```python
from build123d import *

# Parameters (mm, degrees)
BOSS_EXTRUDE1_DEPTH = 3.175
CUT_EXTRUDE1_DEPTH  = 223.25
SKETCH4_W           = 6.35
SKETCH4_H           = 25.4
BOSS_EXTRUDE2_DEPTH = 6.35
LPATTERN1_COUNT     = 3
LPATTERN1_PITCH     = 50.8
SKETCH5_W           = 38.1
SKETCH5_H           = 6.35
BOSS_EXTRUDE3_DEPTH = 6.35
FILLET1_R           = 2.54
CUT_EXTRUDE2_DEPTH  = 6.35


with BuildPart() as part:
    # Sketch1 → Boss-Extrude1 (new, symmetric)
    with BuildSketch(Plane.XY):
        Polygon((0, 190.5), (0, 0), (-114.3, 0), align=None)
    extrude(amount=BOSS_EXTRUDE1_DEPTH, both=True)

    # Sketch2 → Cut-Extrude1 (cut, through all)
    with BuildSketch(Plane.XY.offset(3.175)):
        Polygon((-80.654073281, 19.05), (-19.05, 19.05), (-19.05, 121.723455468), align=None)
    extrude(amount=-CUT_EXTRUDE1_DEPTH, mode=Mode.SUBTRACT)

    # Sketch4 → Boss-Extrude2 (add)
    with BuildSketch(Plane(origin=(0, 0, 0), x_dir=(0, 0, -1), z_dir=(1, 0, 0))):
        with Locations((0, 165.1)):
            Rectangle(SKETCH4_W, SKETCH4_H)
    boss_extrude2 = extrude(amount=BOSS_EXTRUDE2_DEPTH)

    # LPattern1: Boss-Extrude2 ×3
    with Locations(*[(0, -i * LPATTERN1_PITCH, 0) for i in range(1, LPATTERN1_COUNT)]):
        add(boss_extrude2)

    # Sketch5 → Boss-Extrude3 (add)
    with BuildSketch(Plane(origin=(0, 0, 0), x_dir=(-1, 0, 0), z_dir=(0, -1, 0))):
        with Locations((53.975, 0)):
            Rectangle(SKETCH5_W, SKETCH5_H)
    extrude(amount=BOSS_EXTRUDE3_DEPTH)

    # Fillet1
    fillet1_edges = [part.edges().sort_by_distance(p)[0] for p in [
        (-80.654073281, 19.05, 0),
        (-19.05, 121.723455468, 0),
        (-19.05, 19.05, 0),
    ]]
    fillet(fillet1_edges, radius=FILLET1_R)

    # Sketch3 → Cut-Extrude2 (cut)
    with BuildSketch(Plane(origin=(0, 0, -3.175), x_dir=(-1, 0, 0), z_dir=(0, 0, -1))):
        Polygon((91.567, 0), (95.758, 0), (95.758, 8.763), (97.0915, 8.763), (97.0915, 11.303), (95.758, 11.303), (95.758, 14.605), (91.567, 14.605), (91.567, 11.303), (90.2335, 11.303), (90.2335, 8.763), (91.567, 8.763), align=None)
        Polygon((15.367, 0), (19.558, 0), (19.558, 8.763), (20.8915, 8.763), (20.8915, 11.303), (19.558, 11.303), (19.558, 14.605), (15.367, 14.605), (15.367, 11.303), (14.0335, 11.303), (14.0335, 8.763), (15.367, 8.763), align=None)
        Polygon((0, 141.7955), (0, 137.6045), (8.763, 137.6045), (8.763, 136.271), (11.303, 136.271), (11.303, 137.6045), (14.605, 137.6045), (14.605, 141.7955), (11.303, 141.7955), (11.303, 143.129), (8.763, 143.129), (8.763, 141.7955), align=None)
        Polygon((0, 27.4955), (0, 23.3045), (8.763, 23.3045), (8.763, 21.971), (11.303, 21.971), (11.303, 23.3045), (14.605, 23.3045), (14.605, 27.4955), (11.303, 27.4955), (11.303, 28.829), (8.763, 28.829), (8.763, 27.4955), align=None)
    extrude(amount=-CUT_EXTRUDE2_DEPTH, mode=Mode.SUBTRACT)


solid = part.part
```
Read the model definition and answer for the solid it produces. Units are mm, in the model's axes. A direction names the side the tool comes from. Coordinates: 2 decimals unless noted, no trailing zeros. Loops run counter-clockwise (first coordinate to the right, second up) from the corner with the lowest first, then second, coordinate; pieces in that order, holes last.
(1) The mould has two halves that part along Y. Classify faces 1 (the face through (3, 177.8, 0)), 2 (the face through (-73.025, -3, 0)), 3 (the face through (-105, 0, 0)), 4 (the face through (0, 89, 0)): released by +Y, released by -Y, zero draft, split by the parting line, or undercut.
Solution:
face 1: released by +Y
face 2: zero draft
face 3: released by -Y
face 4: undercut
(2) The part is cut by section B-B (y = 97.5). Determine the outline of the cut face in (x, z) (3 decimals), and give its area (3 significant figures).
Solution:
outline: (-55.8, -3.175) - (-33.584, -3.175) - (-33.584, 3.175) - (-55.8, 3.175) - close; (-19.05, -3.175) - (0, -3.175) - (0, 3.175) - (-19.05, 3.175) - close
area: 262 mm2
(3) Consider line 1 along Y through (x, z) = (-4, 1.25); line 2 along X through (y, z) = (5, 1.5); line 3 along Y through (x, z) = (-10, 2.5). Determine where each line is inside the solid, lowest interval first.
Solution:
line 1: y = 0 to 23.3, 27.5 to 137.6, 141.8 to 183.83
line 2: x = -111.3 to -95.76, -91.57 to -19.56, -15.37 to 0
line 3: y = 0 to 21.97, 28.83 to 136.27, 143.13 to 173.83
(4) The part is cut by section D-D (x = -81.5). Determine the outline of the cut face in (y, z) (3 decimals), and give its area (3 significant figures).
Solution:
outline: (0, -3.175) - (54.667, -3.175) - (54.667, 3.175) - (0, 3.175) - close
area: 347 mm2
(5) Flat-ended cylindrical pins translate along their axes: pin 1 Ø1.1 at (y, z) = (23, 0.5) entering from -X; pin 2 Ø3 at (x, z) = (-102.5, 0.5) entering from -Y; pin 3 Ø1.7 at (x, z) = (-13, -1.5) entering from +Y. Find the tip coordinate at first contact, or state that the pin passes through.
Solution:
pin 1: stops at x = -100.83
pin 2: stops at y = 0
pin 3: stops at y = 170.25
(6) The part is cut by section A-A (x = -40.5). Determine the outline of the cut face in (y, z) (3 decimals), and give its area (3 significant figures).
Solution:
outline: (-6.35, -3.175) - (19.05, -3.175) - (19.05, 3.175) - (-6.35, 3.175) - close; (85.973, -3.175) - (123, -3.175) - (123, 3.175) - (85.973, 3.175) - close
area: 396 mm2
(7) A tool of negligible diameter and unlimited length cuts with its end or side. For faces 5 (the face through (-54, -6.35, 0)), 6 (the face through (-4, 137.604, 0)), 7 (the face through (-20.957, 115.013, -0.044)), 8 (the face through (-15.367, 4, 0)), 9 (the face through (-8, 0, 0)), from which of +Z, -Z, +X, -X, +Y, -Y can it reach the whole face along a straight path? Write none if from no direction.
Solution:
face 5: +Z, -Z, +X, -X, -Y
face 6: +Z, -Z, +X
face 7: +Z, -Z
face 8: +Z, -Z, -Y
face 9: +Z, -Z, +X, -Y
(8) The part is cut by section C-C (y = 145.5). Determine the outline of the cut face in (x, z) (3 decimals), and give its area (3 significant figures).
Solution:
outline: (-27, -3.175) - (0, -3.175) - (0, 3.175) - (-27, 3.175) - close
area: 171 mm2
